Check sheet for the modelled part. Datum: model origin and axes. Units: mm. Face numbers are marked on the shaded views. A direction names the side the tool comes from. Coordinates: 2 decimals unless noted, no trailing zeros. Loops run counter-clockwise (first coordinate to the right, second up) from the corner with the lowest first, then second, coordinate; pieces in that order, holes last.
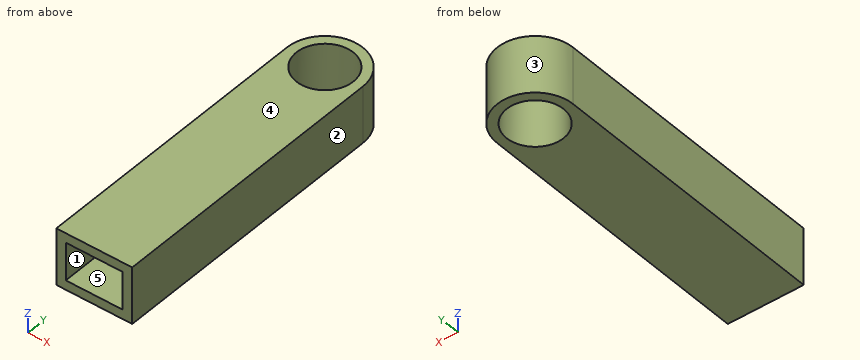
```python
from build123d import *

# Parameters (mm, degrees)
SKETCH_1_R          = 2
SKETCH_1_R_2        = 1.5
EXTRUDE_1_DEPTH     = 3
SKETCH_2_W          = 3
SKETCH_2_H          = 2
CUT_EXTRUDE_1_DEPTH = 10


with BuildPart() as part:
    # 草图1 → 凸台-拉伸1 (new body)
    with BuildSketch(Plane.XY):
        with BuildLine():
            ThreePointArc((2, 0), (0, -2), (-2, 0))
            Line((-2, 0), (-2, -15))
            Line((-2, -15), (2, -15))
            Line((2, -15), (2, 0))
        make_face()
        Circle(SKETCH_1_R)
        Circle(SKETCH_1_R_2, mode=Mode.SUBTRACT)
    extrude(amount=EXTRUDE_1_DEPTH)

    # 草图2 → 切除-拉伸1 (cut)
    with BuildSketch(Plane.XZ.offset(15)):
        with Locations((0, 1.5)):
            Rectangle(SKETCH_2_W, SKETCH_2_H)
    extrude(amount=-CUT_EXTRUDE_1_DEPTH, mode=Mode.SUBTRACT)


solid = part.part
```
1) Section check B-B on y = -11.25. Enter the section's corners in (x, z).
Answer sheet:
outline: (-2, 0) - (2, 0) - (2, 3) - (-2, 3) - close; hole (-1.5, 0.5) - (1.5, 0.5) - (1.5, 2.5) - (-1.5, 2.5) - close
2) Section check D-D on y = 0.5. Enter the section's corners in (x, z).
Answer sheet:
outline: (-1.94, 0) - (-1.41, 0) - (-1.41, 3) - (-1.94, 3) - close; (1.41, 0) - (1.94, 0) - (1.94, 3) - (1.41, 3) - close
3) Section check A-A on x = 0. Enter the section's corners in (y, z), plus the area to 3 significant figures.
Answer sheet:
outline: (-15, 0) - (-1.5, 0) - (-1.5, 3) - (-15, 3) - (-15, 2.5) - (-5, 2.5) - (-5, 0.5) - (-15, 0.5) - close; (1.5, 0) - (2, 0) - (2, 3) - (1.5, 3) - close
area: 22.0 mm2
4) Scan lines: line 1 (Y direction, x = 0.1, z = 2.3); line 2 (X direction, y = -10.25, z = 0.95); line 3 (Z direction, x = 0.95, y = -5.5). Record each from-to range of solid material in increasing order.
Answer sheet:
line 1: y = -5 to -1.5, 1.5 to 2
line 2: x = -2 to -1.5, 1.5 to 2
line 3: z = 0 to 0.5, 2.5 to 3
5) Mould release check, pull along X, two halves, no side actions. Record for the marked faces 3, 4 and 5: +X half, -X half, draft (parallel to the pull), parting line (faces both ways), or undercut.
Answer sheet:
face 3: parting line
face 4: draft
face 5: undercut
6) Depth check by flat-ended pin: pin 1 (1.5 mm diameter, centred on x = 1.5, z = 1.5, fed in from +Y); pin 2 (1 mm diameter, centred on x = 0, y = -8.5, fed in from -Z). Enter the tip coordinate at first touch or a pass-through.
Answer sheet:
pin 1: stops at y = 1.85
pin 2: stops at z = 0
7) Set-up check for the marked faces 1 and 2: record each of +Z, -Z, +X, -X, +Y, -Y from which the full face is reachable in a straight line by a thin tool's end or side.
Answer sheet:
face 1: -Y
face 2: +Z, -Z, +X, +Y, -Y
8) Section check C-C on z = 2.1. Enter the section's corners in (x, y).
Answer sheet:
outline: (-2, -15) - (-1.5, -15) - (-1.5, -5) - (1.5, -5) - (1.5, -15) - (2, -15) - (2, 0) arc R2 ccw to (-2, 0) - close; hole circle Ø3 at (0, 0)
